Verification items for this drawing (mm, ordinates from the low corner). Coordinates: 2 decimals unless noted, no trailing zeros. Loops run counter-clockwise (first coordinate to the right, second up) from the corner with the lowest first, then second, coordinate; pieces in that order, holes last. Notation, with made-up numbers: (15.5, 84.25) - (51.5, 84.25) arc R25 ccw to (51.5, 102.25) - close; hole circle Ø8 at (44, 83.5). An arc over 180 degrees is marked (long way). One line per item, written item: value. Start each with the question number.
(1) Section check B-B (x = 6.35). Count the separate pieces of the cut face and the enclosed holes in it.
(2) Gauge pin test, flat end, axial feed: P1, Ø8, axis at x = 40, z = 13.5, coming from the -Y side (1 decimal). Record the tip position at first contact, or that the pin passes through.
(3) Section check D-D (z = 42.5). Record the boundary of the cut face in (x, y) (1 decimal), plus the area to 3 significant figures.
(4) Thickness scan on probe 1 along Z at (x, y) = (29.5, 15.5) (1 decimal); probe 2 along Y at (x, z) = (6.35, 0.8); probe 3 along Y at (x, z) = (30.5, 54) (1 decimal). Record the ranges inside material, lowest first. Write a range as [from, to].
(5) Section check A-A (y = 47). Record the boundary of the cut face in (x, z) (1 decimal).
(6) Draft check along Z on the marked faces 1, 2, 3 and 4. Enter one of: +Z half, -Z half, draft (parallel to the pull), parting line (faces both ways), or undercut.
(7) Section check C-C (x = 12). Record the boundary of the cut face in (y, z) (1 decimal).
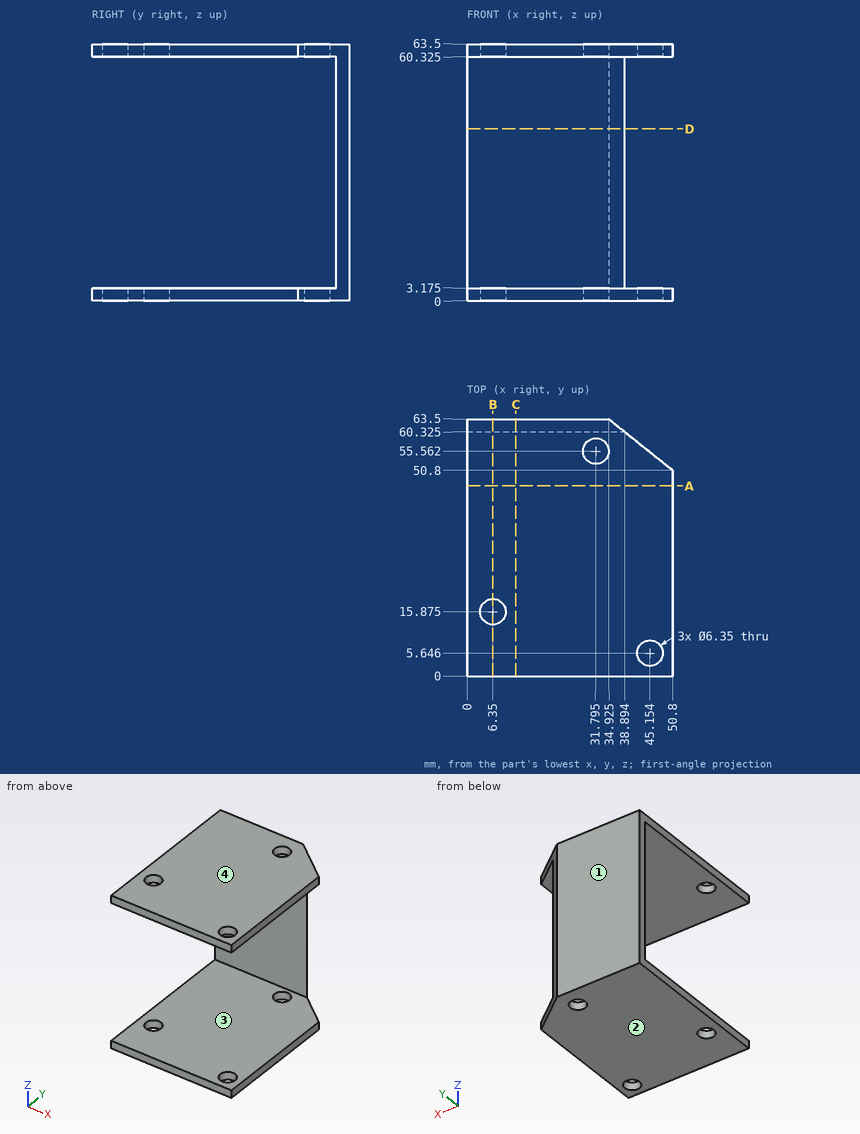
Responses:
1. separate pieces: 3
1. enclosed holes: 0
2. P1: stops at y = 60.3
3. outline: (0, 60.3) - (38.9, 60.3) - (34.9, 63.5) - (0, 63.5) - close
3. area: 117 mm²
4. probe 1: z = [0, 3.2], [60.3, 63.5]
4. probe 2: y = [0, 12.7], [19.05, 63.5]
4. probe 3: y = [60.3, 63.5]
5. outline: (0, 0) - (50.8, 0) - (50.8, 3.2) - (0, 3.2) - close; (0, 60.3) - (50.8, 60.3) - (50.8, 63.5) - (0, 63.5) - close
6. face 1: draft
6. face 2: -Z half
6. face 3: undercut
6. face 4: +Z half
7. outline: (0, 0) - (63.5, 0) - (63.5, 63.5) - (0, 63.5) - (0, 60.3) - (60.3, 60.3) - (60.3, 3.2) - (0, 3.2) - close
